Build history of the part. All positions in model axes, mm. A direction names the side the tool comes from. Give positions to 0.01 mm unless a question says otherwise; leave off trailing zeros. Loops run counter-clockwise (first coordinate to the right, second up) from the corner with the lowest first, then second, coordinate; pieces in that order, holes last. Notation, with made-up numbers: (28, 84) -> (73, 84) arc R18 ccw to (73, 106) -> close; hole circle Ø1 at (73.5, 79). An arc over 180 degrees is marked (long way). Answer as a JSON object with one key per item and string values. Group by question number.
Q1. Band-saw the part on D-D, the plane x = 16. Write the cut outline in (y, z), plus the area to 3 significant figures.
Q2. Tool access for faces 5 (the cylindrical face through (-29.97, 1.32, 23.14)), 6 (the cylindrical face through (159.97, 1.32, 9.86)), 7 (the flat face through (141, 0, 83)): list every direction of +Z, -Z, +X, -X, +Y, -Y with a clear straight run to the whole face (end or side of a thin tool).
Q3. Two-plate mould, pull along X, no slides. Class faces 1 (the cylindrical face through (169.99, 0.88, 16.3)), 2 (the flat face through (0, 0, 13)), 3 (the cylindrical face through (-39.99, -0.88, 16.3)), 4 (the flat face through (64, 40, 16)): pulls with the +X half, pulls with the -X half, needs draft (parallel to the pull), parting line crosses it, or undercut.
Q4. Band-saw the part on B-B, the plane y = 0. Write the cut outline in (x, z).
Q5. Wall check: probe 1 along Y at (x, z) = (130, 16); probe 2 along X at (y, z) = (21, 13.5); probe 3 along Z at (x, y) = (27, 31). Give the ranges that are in metal, low to high. Write a range as from..to.
Q6. Drop flat-ended pins along their axis: pin 1 (3 mm diameter, centred on x = 59, y = -24, fed in from +Z); pin 2 (5 mm diameter, centred on y = 0.5, z = 41, fed in from +X); pin 3 (10 mm diameter, centred on y = -11, z = 67.5, fed in from -X). Give the stop position or say it passes through.
Q7. Band-saw the part on C-C, the plane x = 45. Write the cut outline in (y, z), plus the area to 3 significant figures.
Q8. Band-saw the part on A-A, the plane z = 28. Write the cut outline in (x, y), plus the area to 3 significant figures.
from build123d import *

# Parameters (mm, degrees)
SALIENTE_EXTRUIR1_DEPTH = 33
REDONDEO1_R             = 2.5
CROQUIS2_R              = 30
CORTAR_EXTRUIR1_DEPTH   = 20
CROQUIS3_R              = 30
CORTAR_EXTRUIR2_DEPTH   = 20
CROQUIS4_R              = 19.096631059
SALIENTE_EXTRUIR2_DEPTH = 50
REDONDEO2_R             = 5


with BuildPart() as part:
    # Croquis1 → Saliente-Extruir1 (new body)
    with BuildSketch(Plane.XY):
        with BuildLine():
            Line((0, 40), (130, 40))
            ThreePointArc((130, 40), (170, 0), (130, -40))
            Line((130, -40), (0, -40))
            ThreePointArc((0, -40), (-40, 0), (0, 40))
        make_face()
    extrude(amount=SALIENTE_EXTRUIR1_DEPTH)

    # Redondeo1
    redondeo1_edges = [part.edges().sort_by_distance(p)[0] for p in [
        (170, 0, 33),
        (65, 40, 33),
        (-40, 0, 33),
        (65, 40, 0),
        (170, 0, 0),
        (65, -40, 0),
        (-40, 0, 0),
        (65, -40, 33),
    ]]
    fillet(redondeo1_edges, radius=REDONDEO1_R)

    # Croquis2 → Cortar-Extruir1 (cut)
    with BuildSketch(Plane.XY.offset(33)):
        Circle(CROQUIS2_R)
    extrude(amount=-CORTAR_EXTRUIR1_DEPTH, mode=Mode.SUBTRACT)

    # Croquis3 → Cortar-Extruir2 (cut)
    with BuildSketch(Plane(origin=(0, 0, 0), x_dir=(-1, 0, 0), z_dir=(0, 0, -1))):
        with Locations((-130, 0)):
            Circle(CROQUIS3_R)
    extrude(amount=-CORTAR_EXTRUIR2_DEPTH, mode=Mode.SUBTRACT)

    # Croquis4 → Saliente-Extruir2 (add)
    with BuildSketch(Plane.XY.offset(33)):
        with Locations((140.909108461, 0)):
            Circle(CROQUIS4_R)
    extrude(amount=SALIENTE_EXTRUIR2_DEPTH)

    # Redondeo2
    redondeo2_edges = [part.edges().sort_by_distance(p)[0] for p in [
        (121.812477402, 0, 33),
        (121.812477402, 0, 83),
    ]]
    fillet(redondeo2_edges, radius=REDONDEO2_R)


solid = part.part
Worked answers:
{
 "1": {"outline": "(-40, 2.5) arc R2.5 ccw to (-37.5, 0) -> (37.5, 0) arc R2.5 ccw to (40, 2.5) -> (40, 30.5) arc R2.5 ccw to (37.5, 33) -> (25.38, 33) -> (25.38, 13) -> (-25.38, 13) -> (-25.38, 33) -> (-37.5, 33) arc R2.5 ccw to (-40, 30.5) -> close", "area": "1,620 mm2"},
 "2": {"face 5": "+Z", "face 6": "-Z", "face 7": "+Z, +X, -X, +Y, -Y"},
 "3": {"face 1": "pulls with the +X half", "face 2": "undercut", "face 3": "pulls with the -X half", "face 4": "needs draft"},
 "4": {"outline": "(-40, 2.5) arc R2.5 ccw to (-37.5, 0) -> (100, 0) -> (100, 20) -> (160, 20) -> (160, 0) -> (167.5, 0) arc R2.5 ccw to (170, 2.5) -> (170, 30.5) arc R2.5 ccw to (167.5, 33) -> (165.01, 33) arc R5 cw to (160.01, 38) -> (160.01, 78) arc R5 ccw to (155.01, 83) -> (126.81, 83) arc R5 ccw to (121.81, 78) -> (121.81, 38) arc R5 cw to (116.81, 33) -> (30, 33) -> (30, 13) -> (-30, 13) -> (-30, 33) -> (-37.5, 33) arc R2.5 ccw to (-40, 30.5) -> close"},
 "5": {"probe 1": "-40..-30, 30..40", "probe 2": "-34.04..-21.42, 21.42..108.58, 151.42..164.04", "probe 3": "0..33"},
 "6": {"pin 1": "z = 33", "pin 2": "x = 160.01", "pin 3": "x = 122.78"},
 "7": {"outline": "(-40, 2.5) arc R2.5 ccw to (-37.5, 0) -> (37.5, 0) arc R2.5 ccw to (40, 2.5) -> (40, 30.5) arc R2.5 ccw to (37.5, 33) -> (-37.5, 33) arc R2.5 ccw to (-40, 30.5) -> close", "area": "2,630 mm2"},
 "8": {"outline": "(0, -40) -> (130, -40) arc R40 ccw to (130, 40) -> (0, 40) arc R40 ccw to start; hole circle Ø60 at (0, 0)", "area": "12,600 mm2"}
}
